Build history of the part. All positions in model axes, mm. Face numbers are marked on the shaded views. A direction names the side the tool comes from. Give positions to 0.01 mm unless a question says otherwise; leave off trailing zeros. Order: outer loops, then holes, each group sorted by start corner. A loop starts at its lowest first (then second) coordinate and runs counter-clockwise, first axis right, second up. Notation, with made-up numbers: (56.25, 89.25) - (64.25, 89.25) arc R14 cw to (64.25, 104.25) - close; hole circle Ø7 at (22.5, 32.25). An arc over 180 degrees is marked (long way). Use a Markdown table: item, result.
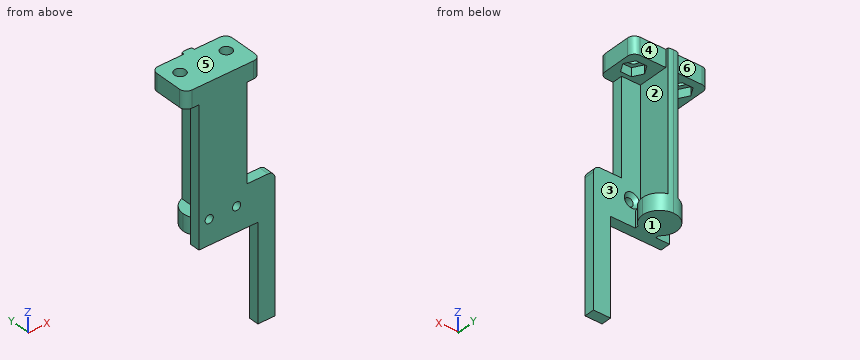
from build123d import *

# Parameters (mm, degrees)
SKETCH1_R                                           = 1.15
BOSS_EXTRUDE1_DEPTH                                 = 3
BOSS_EXTRUDE3_DEPTH                                 = 10
CSK_FOR_M2_COUNTERSUNK_FLAT_HEAD_SCREW2_D           = 2.4
CSK_FOR_M2_COUNTERSUNK_FLAT_HEAD_SCREW2_CSINK_D     = 4.4
CSK_FOR_M2_COUNTERSUNK_FLAT_HEAD_SCREW2_CSINK_ANGLE = 90
CUT_EXTRUDE2_DEPTH                                  = 50.244695146
SKETCH1_4_W                                         = 4
SKETCH1_4_H                                         = 5
SKETCH1_4_W_2                                       = 14
BOSS_EXTRUDE4_DEPTH                                 = 12
SKETCH7_R                                           = 1.65
CUT_EXTRUDE3_DEPTH                                  = 71.880462752
CUT_EXTRUDE4_DEPTH                                  = 2.5
FILLET2_R                                           = 2


with BuildPart() as part:
    # Sketch1 → Boss-Extrude1 (new body)
    with BuildSketch(Plane(origin=(0, 0, 0), x_dir=(1, 0, 0), z_dir=(0, 1, 0))):
        Polygon((7, -6), (15.2, -6), (15.2, 34), (10.2, 34), (10.2, 6), (-7, 6), (-7, -39), (7, -39), align=None)
        with Locations(Location((4, -1.2, 0), (0, 0, 270))):
            Circle(SKETCH1_R, mode=Mode.SUBTRACT)
        with Locations(Location((-4, -1.2, 0), (0, 0, 270))):
            Circle(SKETCH1_R, mode=Mode.SUBTRACT)
    extrude(amount=BOSS_EXTRUDE1_DEPTH)

    # Sketch3 → Boss-Extrude3 (add)
    with BuildSketch(Plane(origin=(0, 3, 0), x_dir=(1, 0, 0), z_dir=(0, 1, 0))):
        Polygon((-5, 1.2), (-1.5, 1.2), (-1.5, -39), (1.5, -39), (1.5, 1.2), (5, 1.2), (5, 6), (-5, 6), align=None)
    extrude(amount=BOSS_EXTRUDE3_DEPTH)

    # CSK for M2 Countersunk Flat Head Screw2 (through all)
    with Locations(Plane(origin=(-4, 3, 1.2), x_dir=(0, 0, 1), z_dir=(0, 1, 0))):
        with Locations((0, 0), (0, 8)):
            CounterSinkHole(CSK_FOR_M2_COUNTERSUNK_FLAT_HEAD_SCREW2_D / 2, CSK_FOR_M2_COUNTERSUNK_FLAT_HEAD_SCREW2_CSINK_D / 2, counter_sink_angle=CSK_FOR_M2_COUNTERSUNK_FLAT_HEAD_SCREW2_CSINK_ANGLE)

    # Sketch6 → Cut-Extrude2 (cut, through all)
    with BuildSketch(Plane(origin=(0, 0, -6), x_dir=(-1, 0, 0), z_dir=(0, 0, -1))):
        with BuildLine():
            Line((-5, 13), (-5, 7.999999988))
            ThreePointArc((-5, 7.999999988), (-3.53553391, 11.535533902), (0, 13))
            Line((0, 13), (-5, 13))
        make_face()
        with BuildLine():
            Line((5, 13), (0, 13))
            ThreePointArc((0, 13), (3.535533906, 11.535533906), (5, 8))
            Line((5, 8), (5, 13))
        make_face()
        with BuildLine():
            Line((5, 3), (5, 8))
            ThreePointArc((5, 8), (4.472135955, 5.763932023), (3, 4))
            Line((3, 4), (3, 3))
            Line((3, 3), (5, 3))
        make_face()
        with BuildLine():
            Line((-5, 3), (-3, 3))
            Line((-3, 3), (-3, 4))
            ThreePointArc((-3, 4), (-4.472135952, 5.763932017), (-5, 7.999999988))
            Line((-5, 7.999999988), (-5, 3))
        make_face()
    extrude(amount=-CUT_EXTRUDE2_DEPTH, mode=Mode.SUBTRACT)

    # Sketch1_4 → Boss-Extrude4 (add)
    with BuildSketch(Plane(origin=(0, 0, 0), x_dir=(1, 0, 0), z_dir=(0, 1, 0))):
        with Locations((-9, -36.5)):
            Rectangle(SKETCH1_4_W, SKETCH1_4_H)
        with Locations((9, -36.5)):
            Rectangle(SKETCH1_4_W, SKETCH1_4_H)
        with Locations((0, -36.5)):
            Rectangle(SKETCH1_4_W_2, SKETCH1_4_H)
    extrude(amount=BOSS_EXTRUDE4_DEPTH)

    # Sketch7 → Cut-Extrude3 (cut, through all)
    with BuildSketch(Plane(origin=(0, 0, 34), x_dir=(-1, 0, 0), z_dir=(0, 0, -1))):
        with Locations((6.75, 7)):
            Circle(SKETCH7_R)
        with Locations(Location((-6.75, 7, 0), (0, 0, 180))):
            Circle(SKETCH7_R)
    extrude(amount=-CUT_EXTRUDE3_DEPTH, mode=Mode.SUBTRACT)

    # Sketch7_3 → Cut-Extrude4 (cut)
    with BuildSketch(Plane(origin=(0, 0, 34), x_dir=(-1, 0, 0), z_dir=(0, 0, -1))):
        Polygon((5.16228676, 9.75), (3.574573519, 7), (5.16228676, 4.25), (8.33771324, 4.25), (9.925426481, 7), (8.33771324, 9.75), align=None)
        Polygon((-5.16228676, 9.75), (-3.574573519, 7), (-5.16228676, 4.25), (-8.33771324, 4.25), (-9.925426481, 7), (-8.33771324, 9.75), align=None)
    extrude(amount=-CUT_EXTRUDE4_DEPTH, mode=Mode.SUBTRACT)

    # Fillet2
    fillet2_edges = [part.edges().sort_by_distance(p)[0] for p in [
        (-11, 12, 36.5),
        (-11, 0, 36.5),
        (11, 12, 36.5),
        (11, 0, 36.5),
        (15.2, 1.5, 6),
    ]]
    fillet(fillet2_edges, radius=FILLET2_R)


solid = part.part
1) Slice it at B-B (z = 20.5). Write the cut outline in (x, y).
Computed:
| item | result |
|---|---|
| outline | (-7, 0) - (7, 0) - (7, 3) - (1.5, 3) - (1.5, 12.77) arc R5 ccw to (-1.5, 12.77) - (-1.5, 3) - (-7, 3) - close |
2) Slice it at C-C (z = -25). Write the cut outline in (x, y), and give its area (3 significant figures).
Computed:
| item | result |
|---|---|
| outline | (10.2, 0) - (15.2, 0) - (15.2, 3) - (10.2, 3) - close |
| area | 15.0 mm² |
3) Two-plate mould, pull along Z, no slides. Class the marked faces 1, 2, 3 and 4: +Z half, -Z half, draft (parallel to the pull), parting line (faces both ways), or undercut.
Computed:
| item | result |
|---|---|
| face 1 | -Z half |
| face 2 | undercut |
| face 3 | undercut |
| face 4 | draft |
4) Tool access for the marked faces 5 and 6: list every direction of +Z, -Z, +X, -X, +Y, -Y with a clear straight run to the whole face (end or side of a thin tool).
Computed:
| item | result |
|---|---|
| face 5 | +Z, +X, -X, +Y, -Y |
| face 6 | +Z, -X, +Y |
5) Slice it at A-A (z = -3.5). Write the cut outline in (x, y).
Computed:
| item | result |
|---|---|
| outline | (-7, 0) - (15.2, 0) - (15.2, 3) - (3, 3) - (3, 4) arc R5 ccw (long way) to (-3, 4) - (-3, 3) - (-7, 3) - close |
6) Wall check: line 1 (X direction, y = 0.75, z = 1.2); line 2 (Y direction, x = 6.75, z = 38.05); line 3 (Z direction, x = -4, y = 1.6). Give the ranges that are in metal, low to high. Write a range as from..to.
Computed:
| item | result |
|---|---|
| line 1 | x = -7..-5.2, -2.8..2.8, 5.2..15.2 |
| line 2 | y = 0..5.35, 8.65..12 |
| line 3 | z = -6..0, 2.4..39 |
7) Pin check, flat tips, straight feed: P1, Ø5, axis at x = -6, y = 3.5, coming from the -Z side; P2, Ø1.2, axis at x = -7, z = 35.5, coming from the +Y side; P3, Ø1.9, axis at x = 4, z = 1.2, coming from the +Y side; P4, Ø0.5, axis at y = 3.5, z = -4, coming from the -X side. Stop position of each tip, or through.
Computed:
| item | result |
|---|---|
| P1 | stops at z = -6 |
| P2 | stops at y = 12 |
| P3 | passes through |
| P4 | stops at x = -3 |
